The model under review builds one solid part; all positions refer to its coordinate system, in mm. Coordinates: 2 decimals unless noted, no trailing zeros. Order: outer loops, then holes, each group sorted by start corner. A loop starts at its lowest first (then second) coordinate and runs counter-clockwise, first axis right, second up. Notation, with made-up numbers: (41, 4.25) -> (100, 4.25) arc R35 ccw to (100, 37.25) -> close; hole circle Ø8 at (-5.5, -4). An arc over 180 degrees is marked (long way). Use one line per item in the form item = value.
from build123d import *

# Parameters (mm, degrees)
SKETCH1_W           = 412.7
SKETCH1_H           = 100
SKETCH1_R           = 4
SKETCH1_R_2         = 5
BOSS_EXTRUDE1_DEPTH = 12.7
CUT_EXTRUDE1_REACH  = 214.701
SKETCH2_R           = 4


with BuildPart() as part:
    # Sketch1 → Boss-Extrude1 (new body)
    with BuildSketch(Plane.XY):
        Rectangle(SKETCH1_W, SKETCH1_H)
        with Locations((-20.590065585, 12.533614425)):
            Circle(SKETCH1_R, mode=Mode.SUBTRACT)
        with Locations((20.590065585, 12.533614425)):
            Circle(SKETCH1_R, mode=Mode.SUBTRACT)
        with Locations((0, -10.30151519)):
            Circle(SKETCH1_R_2, mode=Mode.SUBTRACT)
    extrude(amount=BOSS_EXTRUDE1_DEPTH)

    # Sketch2 → Cut-Extrude1 (cut, up to next)
    with BuildSketch(Plane.XY.offset(12.7), mode=Mode.PRIVATE) as cut_extrude1_sk1:
        with Locations((-180.95, 25)):
            Circle(SKETCH2_R)
    cut_extrude1_tool1 = extrude(cut_extrude1_sk1.sketch, amount=-CUT_EXTRUDE1_REACH, mode=Mode.PRIVATE) & part.part
    # Sketch2 → Cut-Extrude1 (cut, up to next)
    with BuildSketch(Plane.XY.offset(12.7), mode=Mode.PRIVATE) as cut_extrude1_sk2:
        with Locations((-180.95, -25)):
            Circle(SKETCH2_R)
    cut_extrude1_tool2 = extrude(cut_extrude1_sk2.sketch, amount=-CUT_EXTRUDE1_REACH, mode=Mode.PRIVATE) & part.part
    # Sketch2 → Cut-Extrude1 (cut, up to next)
    with BuildSketch(Plane.XY.offset(12.7), mode=Mode.PRIVATE) as cut_extrude1_sk3:
        with Locations((180.95, -25)):
            Circle(SKETCH2_R)
    cut_extrude1_tool3 = extrude(cut_extrude1_sk3.sketch, amount=-CUT_EXTRUDE1_REACH, mode=Mode.PRIVATE) & part.part
    # Sketch2 → Cut-Extrude1 (cut, up to next)
    with BuildSketch(Plane.XY.offset(12.7), mode=Mode.PRIVATE) as cut_extrude1_sk4:
        with Locations((180.95, 25)):
            Circle(SKETCH2_R)
    cut_extrude1_tool4 = extrude(cut_extrude1_sk4.sketch, amount=-CUT_EXTRUDE1_REACH, mode=Mode.PRIVATE) & part.part
    add(cut_extrude1_tool1.solids().sort_by_distance((-180.95, 25, 12.7))[0], mode=Mode.SUBTRACT)
    add(cut_extrude1_tool2.solids().sort_by_distance((-180.95, -25, 12.7))[0], mode=Mode.SUBTRACT)
    add(cut_extrude1_tool3.solids().sort_by_distance((180.95, -25, 12.7))[0], mode=Mode.SUBTRACT)
    add(cut_extrude1_tool4.solids().sort_by_distance((180.95, 25, 12.7))[0], mode=Mode.SUBTRACT)


solid = part.part
Item 1: To check wall thickness, follow L1, parallel to Y at x = -180.95, z = 8.5; L2, parallel to Y at x = 0, z = 7.5; L3, parallel to X at y = -26, z = 8.25. State the ranges of each line that lie inside material, in increasing order. Write a range as from..to.
Results found:
L1 = -50..-29, -21..21, 29..50
L2 = -50..-15.3, -5.3..50
L3 = -206.35..-184.82, -177.08..177.08, 184.82..206.35
Item 2: Clearance check with a flat-ended pin moving along its axis: pin 1 (7 mm diameter, centred on x = 180.95, y = -25, fed in from -Z). State where the tip first meets the part, or that it passes through.
Results found:
pin_1 = through
Item 3: We need section C-C (x = -180.95). Write out the cut boundary in (y, z).
Results found:
outline = (-50, 0) -> (-29, 0) -> (-29, 12.7) -> (-50, 12.7) -> close; (-21, 0) -> (21, 0) -> (21, 12.7) -> (-21, 12.7) -> close; (29, 0) -> (50, 0) -> (50, 12.7) -> (29, 12.7) -> close
Item 4: Draft analysis for pull direction X (two halves, no side actions). For faces 1 (the face through (-3, -50, 6)), 2 (the face through (206.35, -1, 6)), 3 (the face through (176.954, 25.176, 6.439)), state which applies: released by +X, released by -X, zero draft, split by the parting line, or undercut.
Results found:
face_1 = zero draft
face_2 = released by +X
face_3 = undercut
Item 5: We need section B-B (y = 25). Write out the cut boundary in (x, z), plus the area to 3 significant figures.
Results found:
outline = (-206.35, 0) -> (-184.95, 0) -> (-184.95, 12.7) -> (-206.35, 12.7) -> close; (-176.95, 0) -> (176.95, 0) -> (176.95, 12.7) -> (-176.95, 12.7) -> close; (184.95, 0) -> (206.35, 0) -> (206.35, 12.7) -> (184.95, 12.7) -> close
area = 5,040 mm²
Item 6: We need section A-A (x = 0). Write out the cut boundary in (y, z).
Results found:
outline = (-50, 0) -> (-15.3, 0) -> (-15.3, 12.7) -> (-50, 12.7) -> close; (-5.3, 0) -> (50, 0) -> (50, 12.7) -> (-5.3, 12.7) -> close
